from build123d import *

# Parameters (mm, degrees)
SKETCH2_R           = 21.59
BOSS_EXTRUDE1_DEPTH = 144.78
SKETCH3_R           = 19.05
CUT_EXTRUDE1_DEPTH  = 139.7
FILLET1_R           = 21.59
FILLET2_R           = 19.05
SKETCH4_R           = 21.59
CUT_EXTRUDE2_DEPTH  = 17.78


with BuildPart() as part:
    # Sketch2 → Boss-Extrude1 (new body)
    with BuildSketch(Plane(origin=(0, 0, 0), x_dir=(1, 0, 0), z_dir=(0, 1, 0))):
        Circle(SKETCH2_R)
    extrude(amount=BOSS_EXTRUDE1_DEPTH)

    # Sketch3 → Cut-Extrude1 (cut)
    with BuildSketch(Plane.XZ):
        Circle(SKETCH3_R)
    extrude(amount=-CUT_EXTRUDE1_DEPTH, mode=Mode.SUBTRACT)

    # Fillet1
    fillet1_edges = [part.edges().sort_by_distance(p)[0] for p in [
        (-21.59, 144.78, 0),
    ]]
    fillet(fillet1_edges, radius=FILLET1_R)

    # Fillet2
    fillet2_edges = [part.edges().sort_by_distance(p)[0] for p in [
        (-19.05, 139.7, 0),
    ]]
    fillet(fillet2_edges, radius=FILLET2_R)

    # Sketch4 → Cut-Extrude2 (cut)
    with BuildSketch(Plane.XZ):
        Circle(SKETCH4_R)
    extrude(amount=-CUT_EXTRUDE2_DEPTH, mode=Mode.SUBTRACT)


solid = part.part
For this review, take the finished solid that the model builds, in its own axes (mm). Round coordinates to 2 decimals unless told otherwise and drop trailing zeros. Write each loop counter-clockwise with the first axis right and the second up, starting at its lowest first coordinate (ties: lowest second). Pieces come first, ordered by that corner, then holes. Notation, with made-up numbers: M 49,87 L 71,87 A13 ccw 71,108 Z; hole C 79.25,-35 d3. An arc over 180 degrees is marked long. Write item = value, one per line. Start each with the question number.
(1) Clearance check with flat-ended pins moving along their axes: pin 1 Ø4 at (x, y) = (-1, 59.5) entering from -Z; pin 2 Ø12 at (x, y) = (10, 59.5) entering from +Z; pin 3 Ø3 at (x, z) = (2.5, 16.5) entering from +Y. State where each tip first meets the part, or that it passes through.
(2) We need section C-C (y = 116). Give the boundary of the cut face in (x, z), then the cut area to 3 significant figures.
(3) We need section A-A (z = 0). Give the boundary of the cut face in (x, y).
(4) For line 1 along Z through (x, y) = (0, 46); line 2 along Z through (x, y) = (-10, 52); line 3 along X through (y, z) = (66, -5), list the stretches that pass through material, from the lowest coordinate up.
(5) We need section B-B (x = 0). Give the boundary of the cut face in (y, z).
(6) The part is to be moulded in two halves that separate along X. For faces 1 (the face through (-15.913, 69.747, -14.592)), 2 (the face through (-15.12, 68.49, -11.59)), 3 (the face through (7.9, 17.78, -17.5)), say which applies: +X half, -X half, draft (parallel to the pull), parting line (faces both ways), or undercut.
(7) We need section D-D (y = 133.5). Give the boundary of the cut face in (x, z), then the cut area to 3 significant figures.
Results found:
q1.pin_1 = -21.59
q1.pin_2 = 21.22
q1.pin_3 = 138.53
q2.outline = C 0,0 d43.18; hole C 0,0 d38.1
q2.area = 324 mm²
q3.outline = M -21.59,17.78 L -19.05,17.78 L -19.05,120.65 A19.05 cw 19.05,120.65 L 19.05,17.78 L 21.59,17.78 L 21.59,123.19 A21.59 ccw -21.59,123.19 Z
q4.line_1 = -21.59 to -19.05, 19.05 to 21.59
q4.line_2 = -19.13 to -16.21, 16.21 to 19.13
q4.line_3 = -21 to -18.38, 18.38 to 21
q5.outline = M 17.78,-21.59 L 123.19,-21.59 A21.59 ccw 123.19,21.59 L 17.78,21.59 L 17.78,19.05 L 120.65,19.05 A19.05 cw 120.65,-19.05 L 17.78,-19.05 Z
q6.face_1 = parting line
q6.face_2 = undercut
q6.face_3 = draft
q7.outline = C 0,0 d37.94; hole C 0,0 d28.13
q7.area = 509 mm²
